Part model, mm, in its own coordinate system. A direction names the side the tool comes from. Give positions to 0.01 mm unless a question says otherwise; leave off trailing zeros. Write each loop counter-clockwise with the first axis right and the second up, starting at its lowest first coordinate (ties: lowest second). Pieces come first, ordered by that corner, then holes. Notation, with made-up numbers: (50.5, 14.5) - (97.5, 14.5) arc R27 cw to (97.5, 42.5) - close; hole circle Ø2 at (41, 68.25). An arc over 180 degrees is marked (long way). Answer as a JSON object with one key per item and string values. Group by question number.
Autodesk Inventor part; units mm, degrees
ref_plane "YZ Plane" through (0, 0, 0) normal (1, 0, 0) x (0, 1, 0)
ref_plane "XZ Plane" through (0, 0, 0) normal (0, 1, 0) x (-1, 0, 0)
ref_plane "XY Plane" through (0, 0, 0) normal (0, 0, 1) x (1, 0, 0)
sketch "草图1" plane through (0, 0, 0) normal (0, 0, 1) x (1, 0, 0)
  circle A0 centre (0, 0) radius 140
  circle A1 centre (0, 0) radius 132
  line L0 (0, 140) -> (0, -140)
  line L1 (140, 0) -> (-140, 0)
  line L2 (-98.9949, 98.9949) -> (98.9949, -98.9949)
  line L3 (98.9949, 98.9949) -> (-98.9949, -98.9949)
  point P0 (-93.3381, 93.3381)
  point P1 (93.3381, 93.3381)
  dimension "d0" = 280
  dimension "d1" = 8
  dimension "d2" = 90
  dimension "d5" = 45
extrude "拉伸1" add sketch "草图1" along normal blind 10 contours L3 A1 L0 A0 | L0 A1 L2 A0 picked at (81.3579, 110.3999) picked at (-77.3338, 113.2551)
sketch "草图2" plane through (0, 0, 0) normal (0, 0, -1) x (-1, 0, 0)
  circle A0 centre (0, 0) radius 136
  arc A1 (93.3381, 93.3381) -> (-93.3381, 93.3381) centre (0, 0) ccw
  arc A2 (98.9949, 98.9949) -> (-98.9949, 98.9949) centre (0, 0) ccw
  circle A3 centre (91.8302, 100.3155) radius 1.75
  line L0 (98.9949, 98.9949) -> (93.3381, 93.3381)
  line L1 (0, 140) -> (0, 106.7843)
  circle A4 centre (-91.8302, 100.3155) radius 1.75
  dimension "d9" = 4
  dimension "d11" = 3.5
  dimension "d12" = 6
extrude "拉伸2" cut sketch "草图2" against normal blind 29.25 contours A4 A0 | A0 A4 | A3 A0 | A0 A3
sketch "草图3" plane through (0, 0, 0) normal (0, 0, -1) x (-1, 0, 0)
  circle A0 centre (6.4504, 135.8469) radius 1.5
  circle A1 centre (-100.3405, 91.803) radius 1.5
  circle A2 centre (-100.3405, 91.803) radius 1.5
  circle A3 centre (-5.5864, 135.8852) radius 1.5
  circle A4 centre (6.4504, 135.8469) radius 1.25
  circle A5 centre (-5.5864, 135.8852) radius 1.25
  point P0 (0, 0)
  dimension "d27" = 2.5
  dimension "d28" = 2.5
extrude "拉伸3" cut sketch "草图3" against normal blind 29.25 contours A4 | A5
sketch "草图4" plane through (0, 0, 10) normal (0, 0, 1) x (1, 0, 0)
  line L0 (0, 0) -> (-63.3975, 153.0551)
  line L1 (0, 0) -> (0, 175.6772)
  line L2 (0, 0) -> (-105.4105, 105.4105)
  line L3 (-98.9949, 98.9949) -> (-93.3381, 93.3381)
  circle A0 centre (0, 0) radius 135.032
  circle A1 centre (-51.6745, 124.7533) radius 1.5
  circle A2 centre (51.6745, 124.7533) radius 1.5
  circle A3 centre (-51.6745, 124.7533) radius 1.25
  circle A4 centre (51.6745, 124.7533) radius 1.25
  dimension "d23" = 270.064
  dimension "d21" = 22.5
  dimension "d22" = 22.5
  dimension "d24" = 3
  dimension "d33" = 2.5
  dimension "d34" = 2.5
extrude "拉伸4" cut sketch "草图4" against normal blind 10 contours A3 A0 L0 | L0 A0 A3 | A0 A3 L0 | L0 A3 A0 | A4 A0 | A0 A4
thread "螺纹1"
thread "螺纹2"
thread "螺纹3"
thread "螺纹4"
sketch "草图7" plane through (0, 0, 0) normal (0, 0, -1) x (-1, 0, 0)
  circle A0 centre (-91.8302, 100.3155) radius 1.75
  circle A1 centre (-91.8302, 100.3155) radius 2.75
  point P0 (0, 0)
  dimension "d39" = 5.5
extrude "拉伸5" cut sketch "草图7" against normal blind 6 contours A0 | A1
mirror "镜像1" about plane through (0, 0, 0) normal (1, 0, 0) of "拉伸5"
properties part number "组合"
1) Saw through at B-B (z = 1.75). List the corners of the cut face in (x, y), and give its area (3 significant figures).
2) Saw through at D-D (x = -77). List the corners of the cut face in (y, z), and give its area (3 significant figures).
3) Which spindle directions (+Z, -Z, +X, -X, +Y, -Y) get a long thin tool onto all of the face, cutting with end or side? Do faces 1 (the cylindrical face through (-1.451, 131.992, 4.93)), 2 (the cylindrical face through (93.86, 102.17, 2.96)). Say none if no direction does.
4) Saw through at A-A (y = 117.5). List the corners of the cut face in (x, z), and give its area (3 significant figures).
5) Drill centre lines: line 1 along X through (y, z) = (110, 2.75); line 2 along X through (y, z) = (114, 4) (3 decimals); line 3 along X through (y, z) = (100.5, 9.75). Where is each one in solid material? Low to high. Write a range as from..to.
6) Drop flat-ended pins along their axis: P1, Ø3, axis at x = -54, z = 4, coming from the -Y side; P2, Ø6, axis at x = 3, z = 5, coming from the -Y side; P3, Ø1.6, axis at x = -91.5, y = 99, coming from the -Z side. Give the stop position or say it passes through.
7) Saw through at C-C (y = 106.5). List the corners of the cut face in (x, z), and give its area (3 significant figures).
8) Two-plate mould, pull along X, no slides. Class faces 3 (the cylindrical face through (-93.45, 99.65, 7.97)), 4 (the cylindrical face through (-1.54, 139.99, 4.93)), 5 (the flat face through (-96, 96, 5)): +X half, -X half, draft (parallel to the pull), parting line (faces both ways), or undercut.
Checks:
{
 "1": {"outline": "(-98.99, 98.99) - (-93.34, 93.34) arc R132 cw to (93.34, 93.34) - (98.99, 98.99) arc R140 ccw to start; hole circle Ø5.5 at (-91.83, 100.32); hole circle Ø2.5 at (-51.67, 124.75); hole circle Ø2.5 at (-6.45, 135.85); hole circle Ø2.5 at (5.59, 135.89); hole circle Ø2.5 at (51.67, 124.75); hole circle Ø5.5 at (91.83, 100.32)", "area": "1,640 mm2"},
 "2": {"outline": "(107.21, 0) - (116.92, 0) - (116.92, 10) - (107.21, 10) - close", "area": "97.1 mm2"},
 "3": {"face 1": "+Z, -Z, -Y", "face 2": "-Z"},
 "4": {"outline": "(-76.12, 0) - (-60.15, 0) - (-60.15, 10) - (-76.12, 10) - close; (60.15, 0) - (76.12, 0) - (76.12, 10) - (60.15, 10) - close", "area": "319 mm2"},
 "5": {"line 1": "-86.6..-72.97, 72.97..86.6", "line 2": "-81.265..-66.543, 66.543..81.265", "line 3": "-97.47..-93.57, -90.09..-85.58, 85.58..90.09, 93.57..97.47"},
 "6": {"P1": "y = 119.77", "P2": "y = 131.86", "P3": "z = 6"},
 "7": {"outline": "(-90.87, 0) - (-77.99, 0) - (-77.99, 10) - (-90.87, 10) - close; (77.99, 0) - (90.87, 0) - (90.87, 10) - (77.99, 10) - close", "area": "258 mm2"},
 "8": {"face 3": "undercut", "face 4": "parting line", "face 5": "-X half"}
}
